The drawing under review shows one solid part. Ordinate dimensions are in mm from its lowest x, y, z. A direction names the side the tool comes from. Give positions to 0.01 mm unless a question says otherwise; leave off trailing zeros. Write each loop counter-clockwise with the first axis right and the second up, starting at its lowest first coordinate (ties: lowest second). Pieces come first, ordered by that corner, then holes. Notation, with made-up numbers: (9, -11.75) -> (23, -11.75) arc R19 ccw to (23, 17.25) -> close; hole circle Ø1 at (27, 28.5). An arc over 180 degrees is marked (long way). Answer as a JSON object with one key per item and string values.
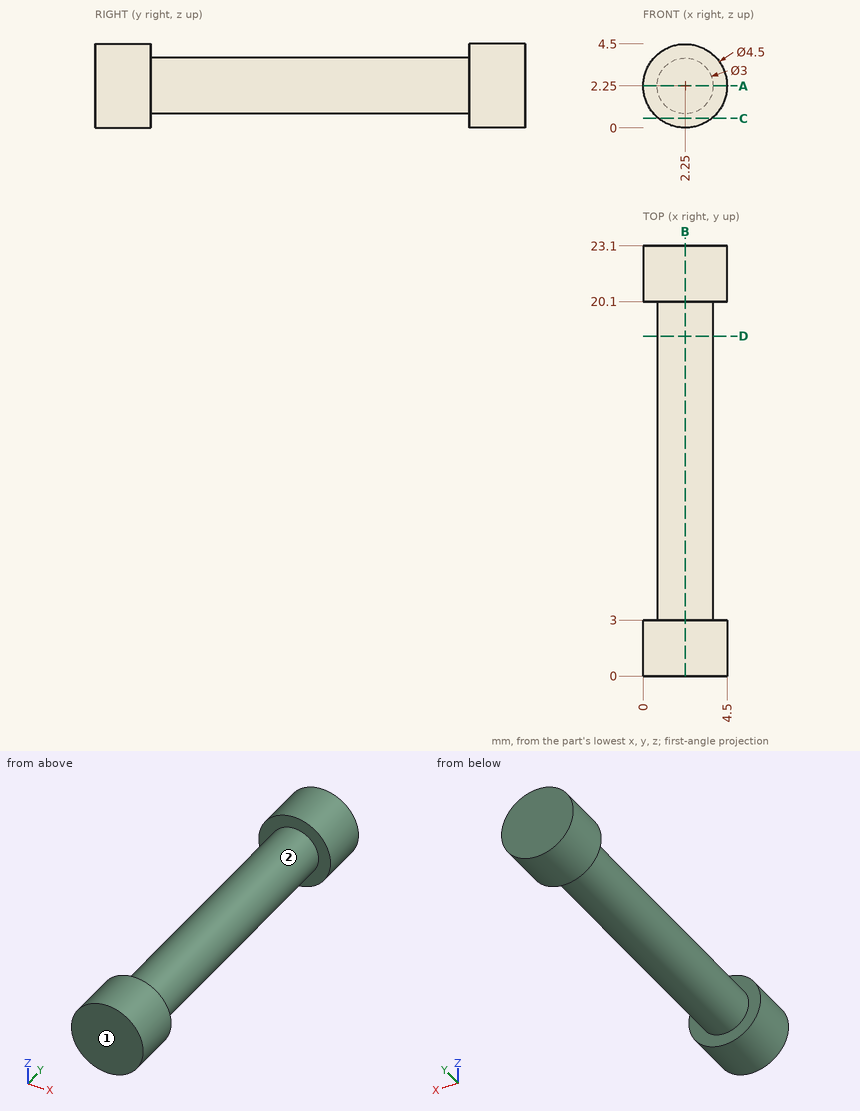
(1) We need section D-D, the plane y = 18.25. State the section outline as (x, z) points, then the cut area to 3 significant figures.
Here are the results:
{"outline": "circle Ø3 at (2.25, 2.25)", "area": "7.07 mm²"}
(2) We need section C-C, the plane z = 0.5. State the section outline as (x, y) points.
Here are the results:
{"outline": "(0.84, 0) -> (3.66, 0) -> (3.66, 3) -> (0.84, 3) -> close; (0.84, 20.1) -> (3.66, 20.1) -> (3.66, 23.1) -> (0.84, 23.1) -> close"}
(3) We need section B-B, the plane x = 2.25. State the section outline as (y, z) points.
Here are the results:
{"outline": "(0, 0) -> (3, 0) -> (3, 0.75) -> (20.1, 0.75) -> (20.1, 0) -> (23.1, 0) -> (23.1, 4.5) -> (20.1, 4.5) -> (20.1, 3.75) -> (3, 3.75) -> (3, 4.5) -> (0, 4.5) -> close"}
(4) We need section A-A, the plane z = 2.25. State the section outline as (x, y) points, then the cut area to 3 significant figures.
Here are the results:
{"outline": "(0, 0) -> (4.5, 0) -> (4.5, 3) -> (3.75, 3) -> (3.75, 20.1) -> (4.5, 20.1) -> (4.5, 23.1) -> (0, 23.1) -> (0, 20.1) -> (0.75, 20.1) -> (0.75, 3) -> (0, 3) -> close", "area": "78.3 mm²"}
(5) For the marked faces 1 and 2, list the 3-axis set-ups (+Z, -Z, +X, -X, +Y, -Y) from which the entire face can be reached by the end or side of a thin tool; tool diameter is ignored.
Here are the results:
{"face 1": "+Z, -Z, +X, -X, -Y", "face 2": "none"}
(6) For line 1 along Y through (x, z) = (2.9, 4.15); line 2 along Z through (x, y) = (2.4, 1.25) (3 decimals); line 3 along X through (y, z) = (16, 2.2), list the stretches that pass through material, from the lowest coordinate up.
Here are the results:
{"line 1": "y = 0 to 3, 20.1 to 23.1", "line 2": "z = 0.005 to 4.495", "line 3": "x = 0.75 to 3.75"}
